Geometry check sheet. Reference: the model listing, model coordinates, mm. A direction names the side the tool comes from. Give positions to 0.01 mm unless a question says otherwise; leave off trailing zeros. Loops run counter-clockwise (first coordinate to the right, second up) from the corner with the lowest first, then second, coordinate; pieces in that order, holes last.
Autodesk Inventor part; units mm, degrees
ref_plane "YZ Plane" through (0, 0, 0) normal (1, 0, 0) x (0, 1, 0)
ref_plane "XZ Plane" through (0, 0, 0) normal (0, 1, 0) x (-1, 0, 0)
ref_plane "XY Plane" through (0, 0, 0) normal (0, 0, 1) x (1, 0, 0)
sketch "Sketch1" plane through (0, 0, 0) normal (0, 1, 0) x (-1, 0, 0)
  circle A0 centre (0, -133.35) radius 1.5875
  line L0 (1.5875, -133.35) -> (-1.5875, -133.35)
  line L1 (-42.8213, -132.9753) -> (-42.8213, -119.5631)
  line L2 (-6.4213, -188.8018) -> (-12.5713, -188.8018)
  line L3 (-6.4213, -194.9518) -> (-6.4213, -188.8018)
  line L4 (-12.5713, -188.8018) -> (-12.5713, -176.1018)
  line L5 (-12.5713, -188.8018) -> (-12.5713, -176.1018)
  line L6 (6.2787, -194.9518) -> (-6.4213, -194.9518)
  line L7 (6.2787, -194.9518) -> (-6.4213, -194.9518)
  line L8 (-12.5713, -176.1018) -> (-6.4213, -176.1018)
  line L9 (6.2787, -188.8018) -> (6.2787, -194.9518)
  line L10 (-6.4213, -176.1018) -> (-6.4213, -169.9518)
  line L11 (-6.4213, -194.9518) -> (-6.4213, -169.9518)
  line L12 (6.2787, -169.9518) -> (6.2787, -194.9518)
  line L13 (-6.4213, -169.9518) -> (6.2787, -169.9518)
  line L14 (-6.4213, -169.9518) -> (6.2787, -169.9518)
  line L15 (-12.5713, -176.1018) -> (12.4167, -176.1018)
  line L16 (12.4167, -188.8018) -> (-12.5713, -188.8018)
  circle A1 centre (-12.5713, -194.9518) radius 1.5875
  line L17 (6.2787, -169.9518) -> (6.2787, -176.1018)
  line L18 (12.4167, -188.8018) -> (6.2787, -188.8018)
  line L19 (6.2787, -176.1018) -> (12.4167, -176.1018)
  line L20 (12.4167, -176.1018) -> (12.4167, -188.8018)
  line L21 (12.4167, -176.1018) -> (12.4167, -188.8018)
  line L22 (0, -169.5003) -> (0, -169.4888)
  circle A2 centre (12.4287, -169.9518) radius 1.5875
  circle A3 centre (-12.5713, -169.9518) radius 1.5875
  circle A4 centre (12.4287, -194.9518) radius 1.5875
  circle A5 centre (-28.1555, -130.3624) radius 1.5875
  line L23 (0, -131.7625) -> (0, -134.9375)
  line L24 (-42.8213, -119.5631) -> (42.8213, -119.5631)
  line L25 (42.8213, -119.5631) -> (42.8213, -209.2768)
  line L26 (39.6463, -212.4518) -> (-39.6463, -212.4518)
  line L27 (-42.8213, -209.2768) -> (-42.8213, -119.5631)
  circle A6 centre (28.1555, -130.3624) radius 1.5875
  arc A7 (39.6463, -212.4518) -> (42.8213, -209.2768) centre (39.6463, -209.2768) ccw
  arc A8 (-42.8213, -209.2768) -> (-39.6463, -212.4518) centre (-39.6463, -209.2768) ccw
  arc A9 (-42.8213, -119.5631) -> (42.8213, -119.5631) centre (0, 0) ccw
  point P0 (-26.811, -129.5183)
  point P1 (-26.811, -129.5183)
  point P2 (26.811, -129.5183)
  point P3 (26.811, -129.5183)
  dimension "d0" = 3.175
  dimension "d2" = 36.6018
  dimension "d4" = 25
  dimension "d6" = 3.175
  dimension "d8" = 3.175
  dimension "d9" = 254
extrude "Extrusion1" add sketch "Sketch1" along normal blind 6.35 contours L1 A9 L25 A7 L26 A8 L27
properties part number "Camera_Mount_Acryllic"
1) Sectioned sample at D-D on x = -16. Enter the section's corners in (y, z).
2) Depth check by flat-ended pin: P1, Ø1.8, axis at x = 10, y = 4.5, coming from the +Z side. Enter the tip coordinate at first touch or a pass-through.
3) Mould release check, pull along Z, two halves, no side actions. Record for faces 3 (the flat face through (-1, 3, -212.452)), 4 (the cylindrical face through (-12.222, 3.131, -171.526)), 5 (the flat face through (1, 0, -165)): +Z half, -Z half, draft (parallel to the pull), parting line (faces both ways), or undercut.
4) Sectioned sample at C-C on y = 1.75. Count the separate pieces of the cut face and the enclosed holes in it, plus the area to 3 significant figures.
5) Sectioned sample at A-A on z = -133.35. Enter the section's corners in (x, y).
6) Scan lines: line 1 along Z through (x, y) = (0, 4.5); line 2 along X through (y, z) = (5.5, -175.5); line 3 along X through (y, z) = (5.5, -131). Record each from-to range of solid material in increasing order.
7) Tool access check on faces 1 (the flat face through (1, 6.35, -165)), 2 (the flat face through (6.421, 3, -192)). Record the directions out of +Z, -Z, +X, -X, +Y, -Y that give a thin tool (end or side, any length) a straight path to the whole face; none if there is none.
8) Sectioned sample at B-B on x = 4.5. Enter the section's corners in (y, z), plus the area to 3 significant figures.
Determined:
1. outline: (0, -212.45) - (6.35, -212.45) - (6.35, -125.99) - (0, -125.99) - close
2. P1: stops at z = -126.53
3. face 3: -Z half
3. face 4: undercut
3. face 5: draft
4. separate pieces: 1
4. enclosed holes: 8
4. area: 6,990 mm2
5. outline: (-42.82, 0) - (-1.59, 0) - (-1.59, 6.35) - (-42.82, 6.35) - close; (1.59, 0) - (42.82, 0) - (42.82, 6.35) - (1.59, 6.35) - close
6. line 1: z = -212.45 to -194.95, -169.95 to -134.94, -131.76 to -127
6. line 2: x = -42.82 to -6.28, 6.42 to 42.82
6. line 3: x = -42.82 to -29.61, -26.7 to 26.7, 29.61 to 42.82
7. face 1: +Z, -Z, +X, -X, +Y
7. face 2: +Y, -Y
8. outline: (0, -212.45) - (6.35, -212.45) - (6.35, -194.95) - (0, -194.95) - close; (0, -169.95) - (6.35, -169.95) - (6.35, -126.92) - (0, -126.92) - close
8. area: 384 mm2
